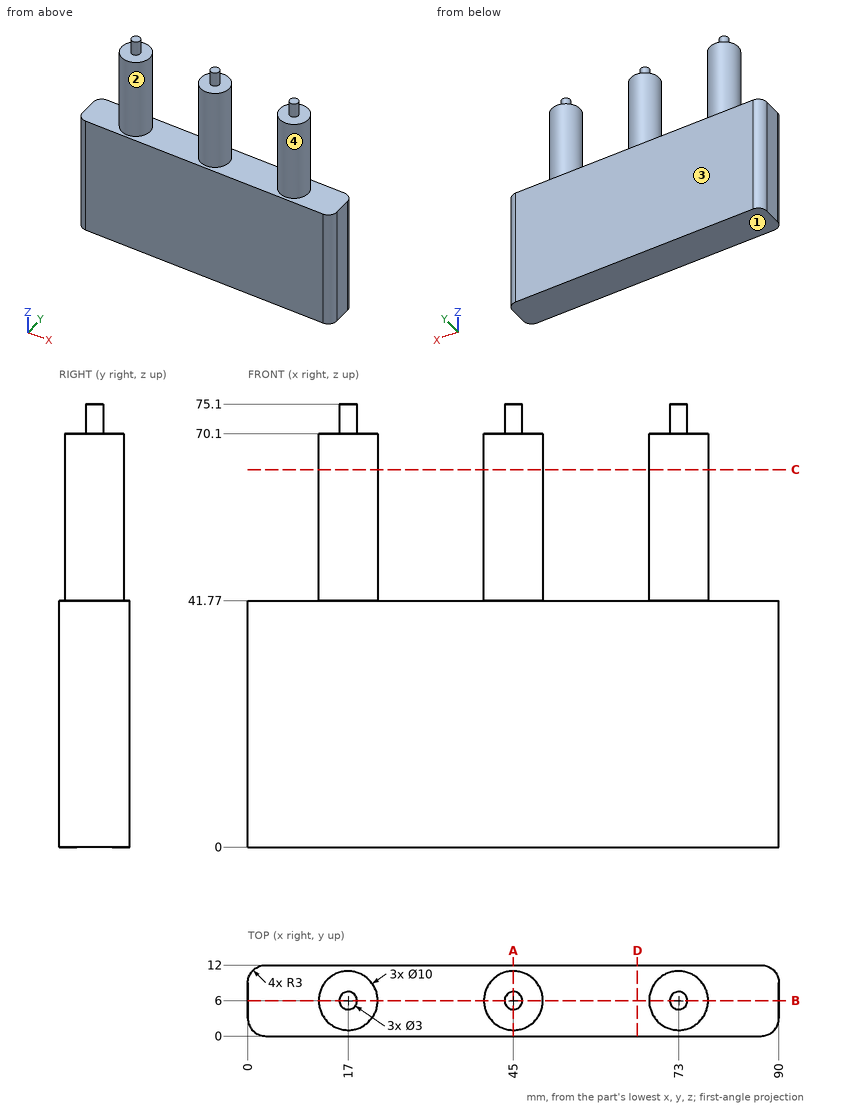
The drawing under review shows one solid part. Ordinate dimensions are in mm from its lowest x, y, z. A direction names the side the tool comes from. Round coordinates to 2 decimals unless told otherwise and drop trailing zeros. Write each loop counter-clockwise with the first axis right and the second up, starting at its lowest first coordinate (ties: lowest second). Pieces come first, ordered by that corner, then holes.
(1) Insertion check: pin 1 (3.5 mm diameter, centred on x = 31.5, y = 6, fed in from +Z); pin 2 (10 mm diameter, centred on x = 56.5, z = 63.5, fed in from +Y). Each pin has a flat end and moves straight along its axis. Give the tip position at first contact, or say it passes through.
(2) We need section D-D on x = 66. Give the boundary of the cut face in (y, z), and give its area (3 significant figures).
(3) We need section C-C on z = 64. Give the boundary of the cut face in (x, y), and give its area (3 significant figures).
(4) We need section B-B on y = 6. Give the boundary of the cut face in (x, z).
(5) Wall thickness on L1, parallel to X at y = 5.5, z = 57; L2, parallel to X at y = 3.5, z = 57; L3, parallel to Z at x = 30, y = 5.5: over which ranges is each line inside the solid? List them lowest first.
(6) Mouldability with a two-part tool opening along X and no side actions: class the marked faces 1 and 2 as +X half, -X half, draft (parallel to the pull), parting line (faces both ways), or undercut.
(7) Machinability: for the marked faces 3 and 4, which of the approach directions +Z, -Z, +X, -X, +Y, -Y give a long, thin tool a straight path to every point of the face, cutting with its end or side? Answer none if there is none.
(8) We need section A-A on x = 45. Give the boundary of the cut face in (y, z), and give its area (3 significant figures).
Findings below:
1. pin 1: stops at z = 41.77
1. pin 2: passes through
2. outline: (0, 0) - (12, 0) - (12, 41.77) - (0, 41.77) - close
2. area: 501 mm2
3. outline: circle Ø10 at (17, 6); circle Ø10 at (45, 6); circle Ø10 at (73, 6)
3. area: 236 mm2
4. outline: (0, 0) - (90, 0) - (90, 41.77) - (78, 41.77) - (78, 70.1) - (74.5, 70.1) - (74.5, 75.1) - (71.5, 75.1) - (71.5, 70.1) - (68, 70.1) - (68, 41.77) - (50, 41.77) - (50, 70.1) - (46.5, 70.1) - (46.5, 75.1) - (43.5, 75.1) - (43.5, 70.1) - (40, 70.1) - (40, 41.77) - (22, 41.77) - (22, 70.1) - (18.5, 70.1) - (18.5, 75.1) - (15.5, 75.1) - (15.5, 70.1) - (12, 70.1) - (12, 41.77) - (0, 41.77) - close
5. L1: x = 12.03 to 21.97, 40.03 to 49.97, 68.03 to 77.97
5. L2: x = 12.67 to 21.33, 40.67 to 49.33, 68.67 to 77.33
5. L3: z = 0 to 41.77
6. face 1: draft
6. face 2: undercut
7. face 3: +Z, -Z, +X, -X, +Y
7. face 4: +Z
8. outline: (0, 0) - (12, 0) - (12, 41.77) - (11, 41.77) - (11, 70.1) - (7.5, 70.1) - (7.5, 75.1) - (4.5, 75.1) - (4.5, 70.1) - (1, 70.1) - (1, 41.77) - (0, 41.77) - close
8. area: 800 mm2
